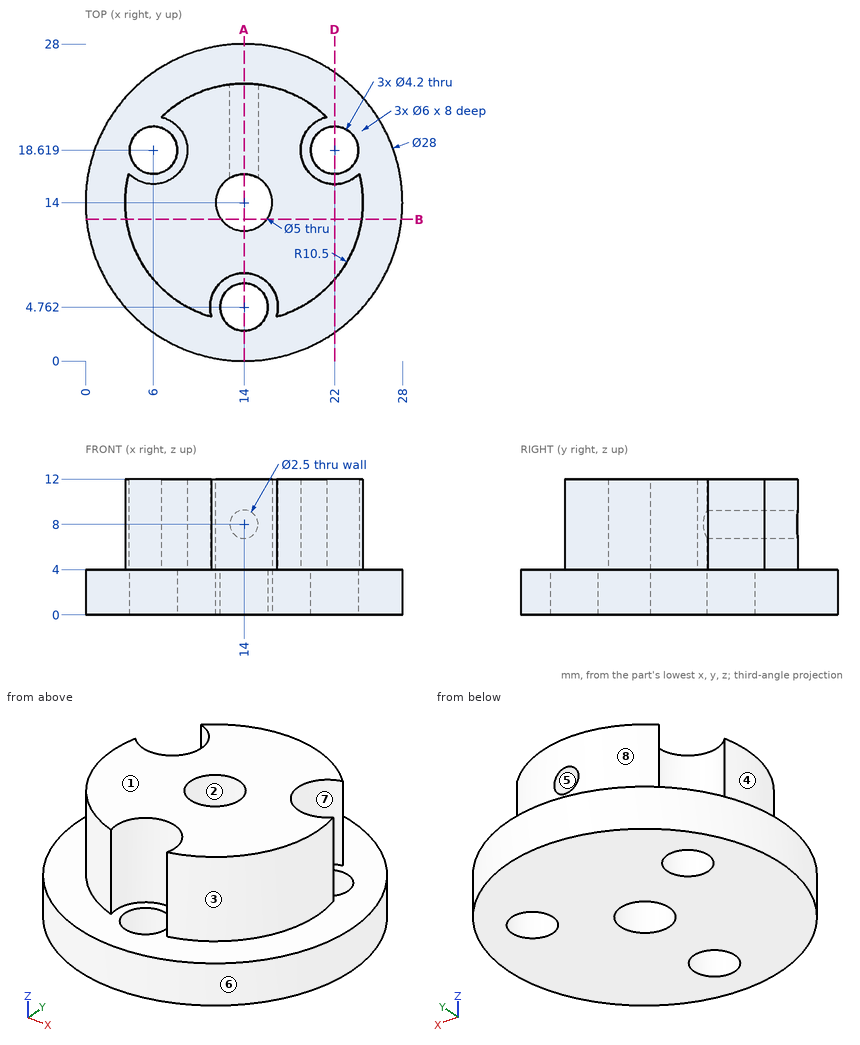
Verification items for this drawing (mm, ordinates from the low corner). A direction names the side the tool comes from. Give positions to 0.01 mm unless a question says otherwise; leave off trailing zeros. Write each loop counter-clockwise with the first axis right and the second up, starting at its lowest first coordinate (ties: lowest second). Pieces come first, ordered by that corner, then holes. Notation, with made-up numbers: (32, 10.25) - (50, 10.25) arc R24 ccw to (50, 22.25) - close; hole circle Ø4 at (79.25, 70). An arc over 180 degrees is marked (long way). Answer as CSV lines item,"result". Start each with the question number.
1. Sectioned sample at B-B (y = 12.5). Record the boundary of the cut face in (x, z).
2. Set-up check for the marked faces 4, 5, 6, 7 and 8: record each of +Z, -Z, +X, -X, +Y, -Y from which the full face is reachable in a straight line by a thin tool's end or side.
3. Sectioned sample at A-A (x = 14). Record the boundary of the cut face in (y, z), then the cut area to 3 significant figures.
4. Sectioned sample at D-D (x = 22). Record the boundary of the cut face in (y, z).
5. Draft check along X on the marked faces 1, 2 and 3. Enter one of: pulls with the +X half, pulls with the -X half, needs draft (parallel to the pull), parting line crosses it, or undercut.
6. Thickness scan on line 1 (X direction, y = 20, z = 2.25); line 2 (X direction, y = 22, z = 7.5) (1 decimal); line 3 (Z direction, x = 5.75, y = 7). Record the ranges inside material, lowest first.
7. Depth check by flat-ended pin: pin 1 (3 mm diameter, centred on x = 14, z = 8, fed in from +Y); pin 2 (3 mm diameter, centred on y = 24.5, z = 7, fed in from -X); pin 3 (2 mm diameter, centred on x = 9, z = 4.5, fed in from -Y) (1 decimal). Enter the tip coordinate at first touch or a pass-through.
Derived:
1,outline,"(0.08, 0) - (12, 0) - (12, 12) - (3.61, 12) - (3.61, 4) - (0.08, 4) - close; (16, 0) - (27.92, 0) - (27.92, 4) - (24.39, 4) - (24.39, 12) - (16, 12) - close"
2,face 4,"+Z, -X"
2,face 5,"+Y"
2,face 6,"+Z, -Z"
2,face 7,"+Z"
2,face 8,"+Z, +Y"
3,outline,"(0, 0) - (2.66, 0) - (2.66, 4) - (0, 4) - close; (6.86, 0) - (11.5, 0) - (11.5, 12) - (7.76, 12) - (7.76, 4) - (6.86, 4) - close; (16.5, 0) - (28, 0) - (28, 4) - (24.5, 4) - (24.5, 6.75) - (16.5, 6.75) - close; (16.5, 9.25) - (24.5, 9.25) - (24.5, 12) - (16.5, 12) - close"
3,area,"149 mm²"
4,outline,"(2.51, 0) - (16.52, 0) - (16.52, 4) - (15.62, 4) - (15.62, 12) - (7.2, 12) - (7.2, 4) - (2.51, 4) - close; (20.72, 0) - (25.49, 0) - (25.49, 4) - (20.72, 4) - close"
5,face 1,"needs draft"
5,face 2,"undercut"
5,face 3,"pulls with the +X half"
6,line 1,"1.35 to 4.42, 7.58 to 20.42, 23.58 to 26.65"
6,line 2,"7.2 to 12.9, 15.1 to 20.8"
6,line 3,"0 to 4"
7,pin 1,"y = 24.5"
7,pin 2,"x = 8.59"
7,pin 3,"y = 0.6"
